from build123d import *

# Parameters (mm, degrees)
F1_DEPTH = 50
F2_DEPTH = 12.5
F3_DEPTH = 2.5
F4_DEPTH = 15
F5_DEPTH = 15
F6_R     = 4
F6_R_2   = 5
F7_DEPTH = 28.3608646168


with BuildPart() as f1:
    # F0 (on Front) → F1 (new body, symmetric)
    with BuildSketch(Plane.XZ):
        with BuildLine():
            Line((30.8374185115, 14.368654698), (-46.5013422072, 14.368654698))
            Line((-46.5013422072, 14.368654698), (-46.5013422072, -7.6422099188))
            ThreePointArc((-46.5013422072, -7.6422099188), (-44.6414702677, -12.1323379793), (-40.1513422072, -13.9922099188))
            Line((-40.1513422072, -13.9922099188), (45.0415951966, -13.9922099188))
            ThreePointArc((45.0415951966, -13.9922099188), (49.5317232571, -12.1323379793), (51.3915951966, -7.6422099188))
            Line((51.3915951966, -7.6422099188), (51.3915951966, 14.368654698))
            Line((51.3915951966, 14.368654698), (30.8374185115, 14.368654698))
        make_face()
    extrude(amount=F1_DEPTH, both=True)

    # F0 (on Front) → F2 (join, symmetric)
    with BuildSketch(Plane.XZ):
        with BuildLine():
            Line((-46.5013422072, 24.9208568856), (-46.5013422072, 14.368654698))
            Line((-46.5013422072, 14.368654698), (30.8374185115, 14.368654698))
            Line((30.8374185115, 14.368654698), (30.8374185115, 29.3047134256))
            ThreePointArc((30.8374185115, 29.3047134256), (31.435925298, 35.0257883198), (35.4166887701, 39.1781888902))
            Line((35.4166887701, 39.1781888902), (43.1814734347, 42.7832674845))
            ThreePointArc((43.1814734347, 42.7832674845), (42.3700127292, 44.9572589365), (41.9035704488, 47.2303930965))
            Line((41.9035704488, 47.2303930965), (-35.384222781, 37.5218286374))
            ThreePointArc((-35.384222781, 37.5218286374), (-43.324802274, 33.3228630958), (-46.5013422072, 24.9208568856))
        make_face()
    extrude(amount=F2_DEPTH, both=True)

    # F0 (on Front) → F3 (join, symmetric)
    with BuildSketch(Plane.XZ):
        with BuildLine():
            Line((30.8374185115, 29.3047134256), (30.8374185115, 14.368654698))
            Line((30.8374185115, 14.368654698), (51.3915951966, 14.368654698))
            Line((51.3915951966, 14.368654698), (55.2041724073, 34.1836406995))
            ThreePointArc((55.2041724073, 34.1836406995), (48.0599839593, 36.8996898007), (43.1814734347, 42.7832674845))
            Line((43.1814734347, 42.7832674845), (35.4166887701, 39.1781888902))
            ThreePointArc((35.4166887701, 39.1781888902), (31.435925298, 35.0257883198), (30.8374185115, 29.3047134256))
        make_face()
    extrude(amount=F3_DEPTH, both=True)

    # F0 (on Front) → F4 (join, symmetric)
    with BuildSketch(Plane.XZ):
        with BuildLine():
            Line((46.8645829495, 47.8535744248), (41.9035704488, 47.2303930965))
            ThreePointArc((41.9035704488, 47.2303930965), (42.3700127292, 44.9572589365), (43.1814734347, 42.7832674845))
            Line((43.1814734347, 42.7832674845), (47.7165182734, 44.8888240168))
            ThreePointArc((47.7165182734, 44.8888240168), (47.1755444697, 46.3381516515), (46.8645829495, 47.8535744248))
        make_face()
    extrude(amount=F4_DEPTH, both=True)

    # F0 (on Front) → F5 (join, symmetric)
    with BuildSketch(Plane.XZ):
        with BuildLine():
            ThreePointArc((43.1814734347, 42.7832674845), (48.0599839593, 36.8996898007), (55.2041724073, 34.1836406995))
            ThreePointArc((55.2041724073, 34.1836406995), (66.8181448931, 37.9478849573), (71.7866079509, 49.0999370813))
            ThreePointArc((71.7866079509, 49.0999370813), (55.8500083917, 64.0706679007), (41.9035704488, 47.2303930965))
            Line((41.9035704488, 47.2303930965), (46.8645829495, 47.8535744248))
            ThreePointArc((46.8645829495, 47.8535744248), (56.1622082448, 59.0804242942), (66.7866079509, 49.0999370813))
            ThreePointArc((66.7866079509, 49.0999370813), (58.9428898464, 39.3351816626), (47.7165182734, 44.8888240168))
            Line((47.7165182734, 44.8888240168), (43.1814734347, 42.7832674845))
        make_face()
    extrude(amount=F5_DEPTH, both=True)

    # F6 (on face) → F7 (cut, through all)
    with BuildSketch(Plane.XY.offset(14.368654698)):
        with Locations((-36.5013422072, 40)):
            Circle(F6_R)
        with Locations((41.3915951966, 40)):
            Circle(F6_R)
        with Locations((-39.3444672227, -40)):
            Circle(F6_R_2)
        with Locations((41.3915951966, -40)):
            Circle(F6_R_2)
    extrude(amount=-F7_DEPTH, mode=Mode.SUBTRACT)


solid = f1.part
The listing builds one solid part. Answer for the finished solid, in the listing's coordinates (mm). A direction names the side the tool comes from. Coordinates: 2 decimals unless noted, no trailing zeros. Write each loop counter-clockwise with the first axis right and the second up, starting at its lowest first coordinate (ties: lowest second). Pieces come first, ordered by that corner, then holes. Notation, with made-up numbers: (9, 78) - (19, 78) arc R20 ccw to (19, 106) - close; hole circle Ø8 at (37.5, 0). An arc over 180 degrees is marked (long way). Return JSON: item names as keys, results as strings.
1. The part is cut by section B-B on y = -40. Determine the outline of the cut face in (x, z).
Final values:
{"outline": "(-46.5, -7.64) arc R6.35 ccw to (-44.34, -12.41) - (-44.34, 14.37) - (-46.5, 14.37) - close; (-34.34, -13.99) - (36.39, -13.99) - (36.39, 14.37) - (-34.34, 14.37) - close; (46.39, -13.85) arc R6.35 ccw to (51.39, -7.64) - (51.39, 14.37) - (46.39, 14.37) - close"}
2. Consider line 1 along X through (y, z) = (-40, -3.5); line 2 along X through (y, z) = (40, 5); line 3 along Y through (x, z) = (-35, -6.5) (3 decimals). Determine where each line is inside the solid, lowest interval first.
Final values:
{"line 1": "-46.5 to -44.34, -34.34 to 36.39, 46.39 to 51.39", "line 2": "-46.5 to -40.5, -32.5 to 37.39, 45.39 to 51.39", "line 3": "-50 to -42.475, -37.525 to 36.292, 43.708 to 50"}
3. The part is cut by section C-C on x = -30. Determine the outline of the cut face in (y, z), then the cut area to 3 significant figures.
Final values:
{"outline": "(-50, -13.99) - (50, -13.99) - (50, 14.37) - (12.5, 14.37) - (12.5, 38.2) - (-12.5, 38.2) - (-12.5, 14.37) - (-50, 14.37) - close", "area": "3,430 mm^2"}
4. Which of the six approach directions +Z, -Z, +X, -X, +Y, -Y give full straight-line access (tool end or side, diameter ignored) to faces 4 (the face through (43, 2.5, 26)), 5 (the face through (30.837, -8, 22)), 6 (the face through (43, -2.5, 26)), 7 (the face through (67, -15, 46)), 8 (the face through (2, -1, -13.992))?
Final values:
{"face 4": "+Y", "face 5": "+X, -Y", "face 6": "-Y", "face 7": "+Z, +X, -X, -Y", "face 8": "-Z, +X, -X, +Y, -Y"}
5. The part is cut by section D-D on y = -4. Determine the outline of the cut face in (x, z) (3 decimals), then the cut area to 3 significant figures.
Final values:
{"outline": "(-46.501, -7.642) arc R6.35 ccw to (-40.151, -13.992) - (45.042, -13.992) arc R6.35 ccw to (51.392, -7.642) - (51.392, 14.369) - (30.837, 14.369) - (30.837, 29.305) arc R8.875 cw to (35.417, 39.178) - (43.181, 42.783) arc R15 ccw (long way) to (41.904, 47.23) - (-35.384, 37.522) arc R12.7 ccw to (-46.501, 24.921) - close; hole circle Ø20 at (56.787, 49.1)", "area": "5,270 mm^2"}
6. The part is cut by section A-A on z = 6.5. Determine the outline of the cut face in (x, y).
Final values:
{"outline": "(-46.5, -50) - (51.39, -50) - (51.39, 50) - (-46.5, 50) - close; hole circle Ø10 at (-39.34, -40); hole circle Ø8 at (-36.5, 40); hole circle Ø10 at (41.39, -40); hole circle Ø8 at (41.39, 40)"}
7. Each of these flat-tipped pins is pushed along its axis until it touches: pin 1 Ø1 at (x, y) = (23.5, -33) entering from +Z; pin 2 Ø6.5 at (y, z) = (-24.5, 2.5) entering from +X; pin 3 Ø9 at (x, z) = (51.5, 55) entering from -Y. Where does it stop, or does it pass through?
Final values:
{"pin 1": "z = 14.37", "pin 2": "x = 51.39", "pin 3": "y = -15"}
8. For a pull along X with two mould halves and no side action, classify faces 1 (the face through (3, 31, 14.369)), 2 (the face through (53.27, -0.04, 24.14)), 3 (the face through (46.87, -0.21, 47.81)) as +X half, -X half, draft (parallel to the pull), parting line (faces both ways), or undercut.
Final values:
{"face 1": "draft", "face 2": "+X half", "face 3": "undercut"}
